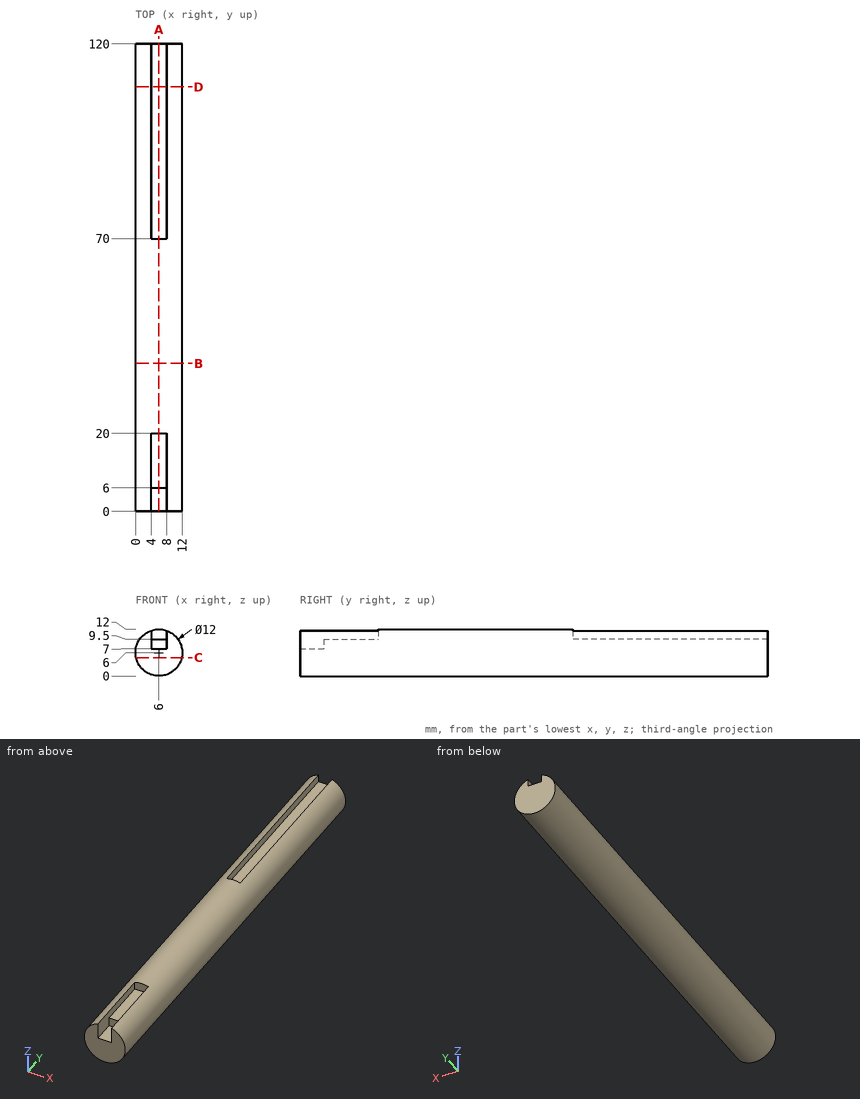
Could you check a few things on this drawing? It's one solid part, dimensions in mm from its lowest x, y, z. Round coordinates to 2 decimals unless told otherwise and drop trailing zeros. Order: outer loops, then holes, each group sorted by start corner. A loop starts at its lowest first (then second) coordinate and runs counter-clockwise, first axis right, second up. Notation, with made-up numbers: M 78.25,-26.5 L 122.25,-26.5 A23 ccw 122.25,9.5 Z; hole C 61,77.25 d4. An arc over 180 degrees is marked long. One line per question, with ' | ' between items.
1) I need wall thicknesses on line 1 (Y direction, x = 5.5, z = 11.75); line 2 (X direction, y = 108, z = 5.75). Which ranges of each line are inside material? Lowest first, please.
Checked values:
line 1: y = 20 to 70 | line 2: x = 0.01 to 11.99
2) Imagine slicing it at A-A, the plane x = 6. Write out the boundary of the cut face in (y, z), plus the area to 3 significant figures.
Checked values:
outline: M 0,0 L 120,0 L 120,9.5 L 70,9.5 L 70,12 L 20,12 L 20,9.5 L 6,9.5 L 6,7 L 0,7 Z | area: 1,250 mm²
3) Imagine slicing it at C-C, the plane z = 4.75. Write out the boundary of the cut face in (x, y).
Checked values:
outline: M 0.13,0 L 11.87,0 L 11.87,120 L 0.13,120 Z
4) Imagine slicing it at D-D, the plane y = 109. Write out the boundary of the cut face in (x, z), plus the area to 3 significant figures.
Checked values:
outline: M 4,9.5 L 4,11.66 A6 ccw long 8,11.66 L 8,9.5 Z | area: 104 mm²
5) I'm going to push flat-ended pins straight in: pin 1 Ø0.6 at (y, z) = (85, 10.5) entering from -X; pin 2 Ø5 at (y, z) = (104.5, 2) entering from -X; pin 3 Ø1.5 at (x, y) = (1.5, 98.5) entering from +Z. Where does each tip first touch, or does it pass through?
Checked values:
pin 1: stops at x = 1.72 | pin 2: stops at x = 0.19 | pin 3: stops at z = 10.68
6) Imagine slicing it at B-B, the plane y = 38. Write out the boundary of the cut face in (x, z), plus the area to 3 significant figures.
Checked values:
outline: C 6,6 d12 | area: 113 mm²
